Geometry: final body of the model. Coordinates: model frame, mm. Round coordinates to 2 decimals unless told otherwise and drop trailing zeros. Loops run counter-clockwise (first coordinate to the right, second up) from the corner with the lowest first, then second, coordinate; pieces in that order, holes last. Notation, with made-up numbers: M 13.25,33 L 60.25,33 A10 cw 60.25,52 Z; hole C 10.25,83 d9. An arc over 180 degrees is marked long. Answer as a JSON object with one key per item and string values.
from build123d import *

# Parameters (mm, degrees)
CROQUIS1_W              = 12.2
CROQUIS1_H              = 22.5
SALIENTE_EXTRUIR1_DEPTH = 3
CROQUIS2_R              = 2.38125
CORTAR_EXTRUIR1_DEPTH   = 4


with BuildPart() as part:
    # Croquis1 → Saliente-Extruir1 (new body)
    with BuildSketch(Plane.XY):
        Polygon((75, 0), (-75, 0), (-150, 0), (-150, 30), (-150, 55), (-120, 55), (-120, 30), (-60, 30), (0, 150), align=None)
        with Locations((-135, 30)):
            Rectangle(CROQUIS1_W, CROQUIS1_H, mode=Mode.SUBTRACT)
    extrude(amount=SALIENTE_EXTRUIR1_DEPTH)

    # Croquis2 → Cortar-Extruir1 (cut, through all)
    with BuildSketch(Plane.XY):
        with Locations((0, 128)):
            Circle(CROQUIS2_R)
        Polygon((5, 140), (0, 150), (-5, 140), align=None)
    extrude(amount=CORTAR_EXTRUIR1_DEPTH, mode=Mode.SUBTRACT)


solid = part.part
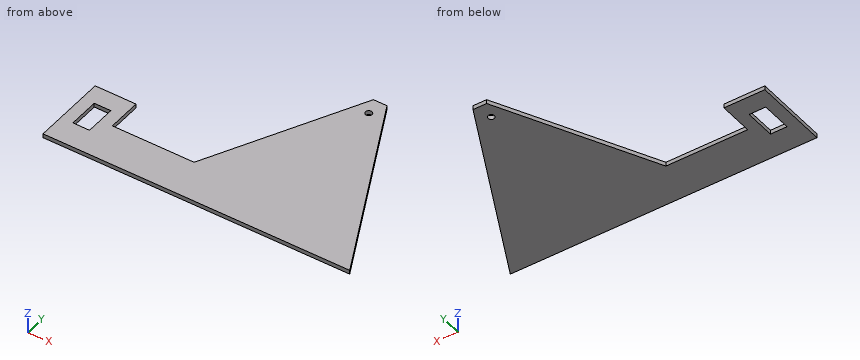
1) Section query D-D (x = -74). Return the cut outline in (y, z), and give its area (3 significant figures).
Results:
{"outline": "M 0,0 L 30,0 L 30,3 L 0,3 Z", "area": "90.0 mm2"}
2) Pin query (flat end, axial travel): P1, Ø0.9, axis at x = -135.5, z = 2, coming from the +Y side; P2, Ø3, axis at x = 0, y = 128, coming from the -Z side; P3, Ø1.5, axis at y = 48.5, z = 2, coming from the +X side (3 decimals); P4, Ø1.5, axis at y = 99, z = 2, coming from the -X side (3 decimals). Return the tip coordinate at first contact, or that it passes through.
Results:
{"P1": "y = 55", "P2": "through", "P3": "x = 51.125", "P4": "x = -25.875"}
3) Section query C-C (y = 128). Return the cut outline in (x, z).
Results:
{"outline": "M -11,0 L -2.38,0 L -2.38,3 L -11,3 Z; M 2.38,0 L 11,0 L 11,3 L 2.38,3 Z"}
4) Section query A-A (x = 0). Return the cut outline in (y, z), and give its area (3 significant figures).
Results:
{"outline": "M 0,0 L 125.62,0 L 125.62,3 L 0,3 Z; M 130.38,0 L 140,0 L 140,3 L 130.38,3 Z", "area": "406 mm2"}
5) Ray query, line 1 (Y direction, x = 0, z = 1.8); line 2 (X direction, y = 128, z = 1.4); line 3 (Y direction, x = -1, z = 1). Return the intervals inside material, ascending.
Results:
{"line 1": "0 to 125.62, 130.38 to 140", "line 2": "-11 to -2.38, 2.38 to 11", "line 3": "0 to 125.84, 130.16 to 140"}
6) Section query B-B (z = 0.9). Return the cut outline in (x, y).
Results:
{"outline": "M -150,0 L 75,0 L 5,140 L -5,140 L -60,30 L -120,30 L -120,55 L -150,55 Z; hole M -141.1,18.75 L -128.9,18.75 L -128.9,41.25 L -141.1,41.25 Z; hole C 0,128 d4.76"}
